from build123d import *

# Parameters (mm, degrees)
F0_R     = 25.4
F0_R_2   = 19.4
F1_DEPTH = 50.8
F2_R     = 3
F3_R     = 0.4
F4_R     = 1


with BuildPart() as f1:
    # F0 (on Top) → F1 (new body)
    with BuildSketch(Plane.XY):
        Circle(F0_R)
        Circle(F0_R_2, mode=Mode.SUBTRACT)
    extrude(amount=F1_DEPTH)

    # F2
    f2_edges = [f1.edges().sort_by_distance(p)[0] for p in [
        (-25.4, 0, 0),
    ]]
    fillet(f2_edges, radius=F2_R)

    # F3
    f3_edges = [f1.edges().sort_by_distance(p)[0] for p in [
        (-25.4, 0, 50.8),
        (-19.4, 0, 0),
    ]]
    fillet(f3_edges, radius=F3_R)

    # F4
    f4_edges = [f1.edges().sort_by_distance(p)[0] for p in [
        (-19.4, 0, 50.8),
    ]]
    fillet(f4_edges, radius=F4_R)


solid = f1.part
Can you work these out from the model? Positions are in its coordinate system, mm. Coordinates: 2 decimals unless noted, no trailing zeros. Write each loop counter-clockwise with the first axis right and the second up, starting at its lowest first coordinate (ties: lowest second). Pieces come first, ordered by that corner, then holes. Notation, with made-up numbers: (32.25, 77.25) - (44.25, 77.25) arc R26 cw to (44.25, 98.25) - close; hole circle Ø10 at (22.25, -12). An arc over 180 degrees is marked (long way). Return JSON: item names as keys, results as strings. Group by question number.
Item 1: If we section it at A-A (y = 0): Write out the boundary of the cut face in (x, z), then the cut area to 3 significant figures.
Item 2: I'm going to push flat-ended pins straight in: pin 1 Ø8 at (y, z) = (19.5, 7) entering from -X; pin 2 Ø3 at (x, z) = (12.5, 19.5) entering from -Y; pin 3 Ø4 at (y, z) = (-10.5, 43) entering from +X. Where does each tip first touch, or does it pass through?
Item 3: We'd pull the mould along X, two halves only. Please class faces 1 (the face through (-9.4, -18.4, 50.8)), 2 (the face through (18.504, 5.827, 24.754)), 3 (the face through (-5.506, -24.796, 26.368)): pulls with the +X half, pulls with the -X half, needs draft (parallel to the pull), parting line crosses it, or undercut.
Item 4: If we section it at C-C (z = 27): Write out the boundary of the cut face in (x, y).
Item 5: Please list where these lines run through material, in increasing order: probe 1 along Y at (x, z) = (0, 26.5); probe 2 along X at (y, z) = (-0.5, 38.5); probe 3 along X at (y, z) = (-16, 31).
Return value:
{
 "1": {"outline": "(-25.4, 3) arc R3 ccw to (-22.4, 0) - (-19.8, 0) arc R0.4 ccw to (-19.4, 0.4) - (-19.4, 49.8) arc R1 ccw to (-20.4, 50.8) - (-25, 50.8) arc R0.4 ccw to (-25.4, 50.4) - close; (19.4, 0.4) arc R0.4 ccw to (19.8, 0) - (22.4, 0) arc R3 ccw to (25.4, 3) - (25.4, 50.4) arc R0.4 ccw to (25, 50.8) - (20.4, 50.8) arc R1 ccw to (19.4, 49.8) - close", "area": "605 mm^2"},
 "2": {"pin 1": "stops at x = -20.12", "pin 2": "stops at y = -22.89", "pin 3": "stops at x = 23.94"},
 "3": {"face 1": "needs draft", "face 2": "undercut", "face 3": "parting line crosses it"},
 "4": {"outline": "circle Ø50.8 at (0, 0); hole circle Ø38.8 at (0, 0)"},
 "5": {"probe 1": "y = -25.4 to -19.4, 19.4 to 25.4", "probe 2": "x = -25.4 to -19.39, 19.39 to 25.4", "probe 3": "x = -19.73 to -10.97, 10.97 to 19.73"}
}
